Source: three-view drawing plus pictorial views. Frame: mm from the lowest corner of the part. A direction names the side the tool comes from. Give positions to 0.01 mm unless a question says otherwise; leave off trailing zeros. Order: outer loops, then holes, each group sorted by start corner. A loop starts at its lowest first (then second) coordinate and runs counter-clockwise, first axis right, second up.
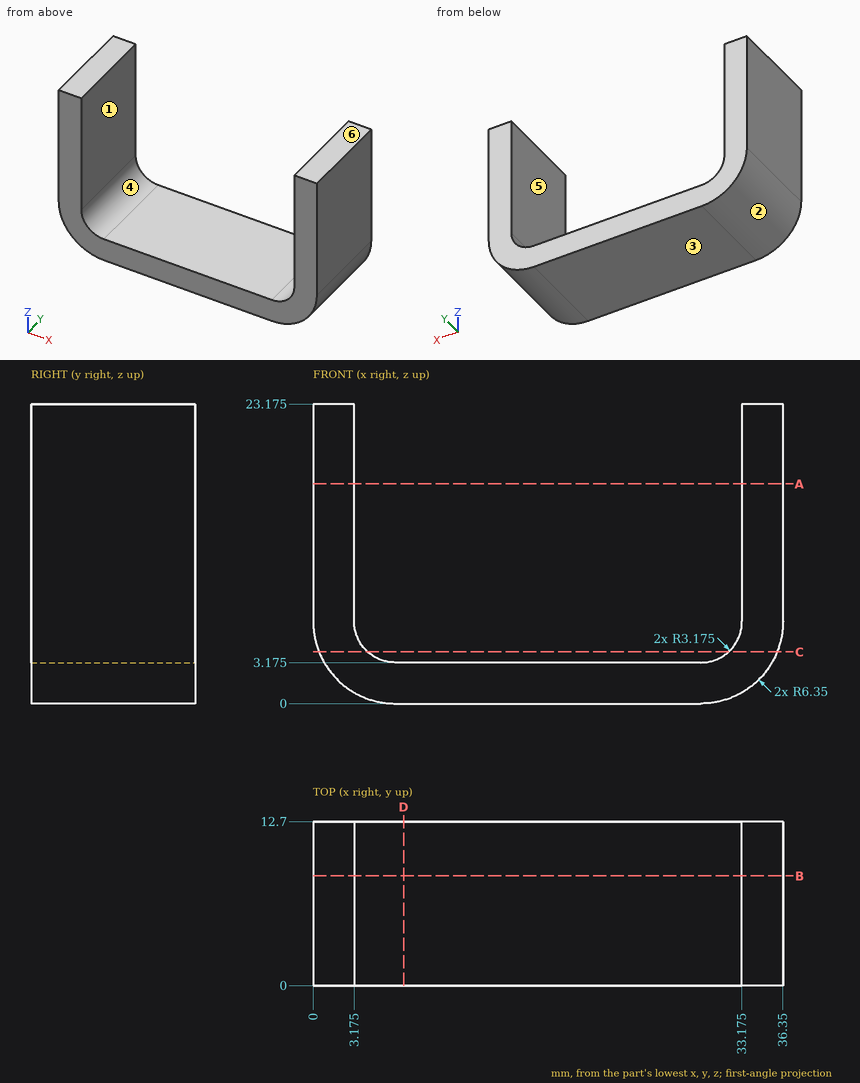
1) Section query C-C on z = 4. Output: boundary loops of the cut face in (x, y).
Checks:
outline: (0.45, 0) - (4.22, 0) - (4.22, 12.7) - (0.45, 12.7) - close; (32.13, 0) - (35.9, 0) - (35.9, 12.7) - (32.13, 12.7) - close
2) Pull-direction query (X, two-part tool) for the marked faces 1, 2, 3 and 4; classes: +X half, -X half, draft (parallel to the pull), parting line (faces both ways), or undercut.
Checks:
face 1: undercut
face 2: -X half
face 3: draft
face 4: undercut
3) Reachability of the marked faces 5 and 6 from +Z, -Z, +X, -X, +Y, -Y: full face, straight path, thin tool, end or side. Return the list, or none.
Checks:
face 5: +Z, +Y, -Y
face 6: +Z, +X, -X, +Y, -Y
4) Section query A-A on z = 17. Output: boundary loops of the cut face in (x, y) (3 decimals).
Checks:
outline: (0, 0) - (3.175, 0) - (3.175, 12.7) - (0, 12.7) - close; (33.175, 0) - (36.35, 0) - (36.35, 12.7) - (33.175, 12.7) - close
5) Ray query, L1, parallel to X at y = 6.25, z = 10.5 (3 decimals); L2, parallel to Z at x = 22.5, y = 9.25 (3 decimals); L3, parallel to X at y = 9.5, z = 4.25. Return the intervals inside material, ascending.
Checks:
L1: x = 0 to 3.175, 33.175 to 36.35
L2: z = 0 to 3.175
L3: x = 0.36 to 3.97, 32.38 to 35.99
6) Section query D-D on x = 7. Output: boundary loops of the cut face in (y, z) (3 decimals), and give its area (3 significant figures).
Checks:
outline: (0, 0) - (12.7, 0) - (12.7, 3.175) - (0, 3.175) - close
area: 40.3 mm2
7) First-contact query: pin 1 Ø4 at (x, y) = (20, 8.5) entering from +Z (3 decimals); pin 2 Ø6 at (x, z) = (31.5, 13.5) entering from -Y; pin 3 Ø12 at (x, z) = (24, 14) entering from +Y. Flat tips, straight axial feed; report the tip coordinate or a pass-through.
Checks:
pin 1: stops at z = 3.175
pin 2: stops at y = 0
pin 3: passes through
8) Section query B-B on y = 8.5. Output: boundary loops of the cut face in (x, z) (3 decimals), and give its area (3 significant figures).
Checks:
outline: (0, 6.35) arc R6.35 ccw to (6.35, 0) - (30, 0) arc R6.35 ccw to (36.35, 6.35) - (36.35, 23.175) - (33.175, 23.175) - (33.175, 6.35) arc R3.175 cw to (30, 3.175) - (6.35, 3.175) arc R3.175 cw to (3.175, 6.35) - (3.175, 23.175) - (0, 23.175) - close
area: 229 mm2
